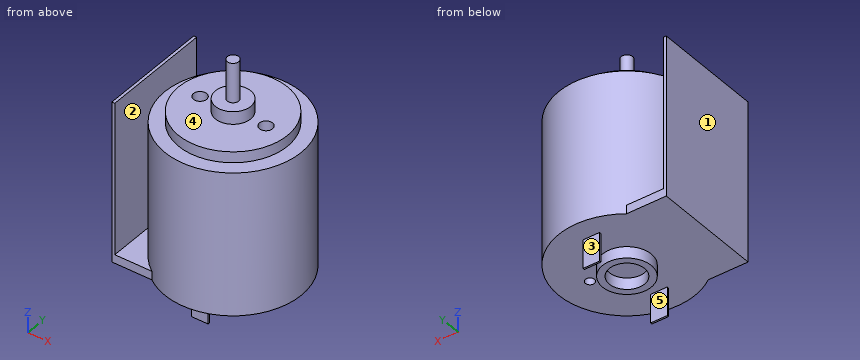
from build123d import *

# Parameters (mm, degrees)
SKETCH_2_R             = 1
EXTRUDE_1_DEPTH        = 36
SKETCH_2_4_R           = 3.075
SKETCH_2_4_R_2         = 1
EXTRUDE_2_DEPTH        = 29.1
EXTRUDE_3_DEPTH        = 26.9
EXTRUDE_3_DEPTH_BACK   = 2
SKETCH_2_5_R           = 4.25
SKETCH_2_5_R_2         = 3.075
SKETCH_2_6_R           = 9.5
SKETCH_2_6_R_2         = 4.25
EXTRUDE_4_DEPTH        = 26.9
SKETCH_2_7_R           = 11.9
SKETCH_2_7_R_2         = 9.5
EXTRUDE_5_DEPTH        = 25
SKETCH_5_W             = 2.9
SKETCH_5_H             = 0.3
EXTRUDE_6_DEPTH        = 5
HOLE_WIZARD_M2_2_D     = 1.6
HOLE_WIZARD_M2_2_DEPTH = 6
HOLE_WIZARD_M2_2_TIP   = 0.480688495
SKETCH_14_R            = 1.15
CUT_EXTRUDE_1_DEPTH    = 3
SKETCH_15_W            = 0.5
SKETCH_15_H            = 19.17801297
EXTRUDE_7_DEPTH        = 28
SKETCH_17_W            = 1.5
SKETCH_17_H            = 19.17801297
EXTRUDE_9_DEPTH        = 10


with BuildPart() as part:
    # Sketch 2 → Extrude 1 (new body)
    with BuildSketch(Plane.XY):
        Circle(SKETCH_2_R)
    extrude(amount=EXTRUDE_1_DEPTH)

    # Sketch 2_4 → Extrude 2 (add)
    with BuildSketch(Plane.XY):
        Circle(SKETCH_2_4_R)
        Circle(SKETCH_2_4_R_2, mode=Mode.SUBTRACT)
    extrude(amount=EXTRUDE_2_DEPTH)

    # Sketch 2_5 → Extrude 3 (add, two sides: drawn at the far end of the back side and taken through both)
    with BuildSketch(Plane.XY.offset(-EXTRUDE_3_DEPTH_BACK)):
        Circle(SKETCH_2_5_R)
        Circle(SKETCH_2_5_R_2, mode=Mode.SUBTRACT)
    extrude(amount=EXTRUDE_3_DEPTH + EXTRUDE_3_DEPTH_BACK)

    # Sketch 2_6 → Extrude 4 (add)
    with BuildSketch(Plane.XY):
        with Locations(Location((0, 0, 0), (0, 0, 180))):
            Circle(SKETCH_2_6_R)
        Circle(SKETCH_2_6_R_2, mode=Mode.SUBTRACT)
    extrude(amount=EXTRUDE_4_DEPTH)

    # Sketch 2_7 → Extrude 5 (add)
    with BuildSketch(Plane.XY):
        Circle(SKETCH_2_7_R)
        with Locations(Location((0, 0, 0), (0, 0, 180))):
            Circle(SKETCH_2_7_R_2, mode=Mode.SUBTRACT)
    extrude(amount=EXTRUDE_5_DEPTH)

    # Sketch 5 → Extrude 6 (add)
    with BuildSketch(Plane(origin=(0, 0, 0), x_dir=(-1, 0, 0), z_dir=(0, 0, -1))):
        with Locations((0, -7.656829655)):
            Rectangle(SKETCH_5_W, SKETCH_5_H)
        with Locations((0, 8.189714354)):
            Rectangle(SKETCH_5_W, SKETCH_5_H)
    extrude(amount=EXTRUDE_6_DEPTH)

    # Hole Wizard M2 _2
    with Locations(Plane(origin=(0, 0, 0), x_dir=(-1, 0, 0), z_dir=(0, 0, -1))):
        with Locations((-6.45, 0), (6.45, 0)):
            Hole(HOLE_WIZARD_M2_2_D / 2, depth=HOLE_WIZARD_M2_2_DEPTH)
            with Locations((0, 0, -(HOLE_WIZARD_M2_2_DEPTH + HOLE_WIZARD_M2_2_TIP / 2))):  # 118° drill point
                Cone(0, HOLE_WIZARD_M2_2_D / 2, HOLE_WIZARD_M2_2_TIP, mode=Mode.SUBTRACT)

    # Sketch 14 → Cut-Extrude 1 (cut)
    with BuildSketch(Plane.XY.offset(26.9)):
        with Locations((5.75, 0)):
            Circle(SKETCH_14_R)
        with Locations((-5.75, 0)):
            Circle(SKETCH_14_R)
    extrude(amount=-CUT_EXTRUDE_1_DEPTH, mode=Mode.SUBTRACT)



with BuildPart() as body_2:
    # Sketch 15 → Extrude 7 (new body)
    with BuildSketch(Plane(origin=(0, 0, 0), x_dir=(-1, 0, 0), z_dir=(0, 0, -1))):
        with Locations((13.75, 0)):
            Rectangle(SKETCH_15_W, SKETCH_15_H)
    extrude(amount=-EXTRUDE_7_DEPTH)


with BuildPart() as part_1:
    add(part.part)

    add(body_2.part)  # Extrude 9 merges body 2
    # Sketch 17 → Extrude 9 (add)
    with BuildSketch(Plane.ZY.offset(14)):
        with Locations((0.75, 0)):
            Rectangle(SKETCH_17_W, SKETCH_17_H)
    extrude(amount=-EXTRUDE_9_DEPTH)


solid = part_1.part
Geometry: final body of the model. Coordinates: model frame, mm. Face numbers are marked on the shaded views. A direction names the side the tool comes from. Round coordinates to 2 decimals unless told otherwise and drop trailing zeros. Loops run counter-clockwise (first coordinate to the right, second up) from the corner with the lowest first, then second, coordinate; pieces in that order, holes last.
Q1. Section C-C on x = -8.5. Return loops of the section in (y, z), plus the area to 3 significant figures.
Q2. Pin query (flat end, axial travel): P1, Ø5, axis at x = -7, z = 25, coming from the +Y side; P2, Ø1.4, axis at x = 0, z = -1.5, coming from the -Y side; P3, Ø3, axis at y = -7.5, z = 8.5, coming from the +X side. Return the tip coordinate at first contact, or that it passes through.
Q3. Section A-A on z = 19.5. Return loops of the section in (x, y), plus the area to 3 significant figures.
Q4. Material intervals for L1, parallel to X at y = 0, z = 2.75; L2, parallel to Y at x = 0, z = -1 (3 decimals); L3, parallel to Z at x = -5.5, y = -6, sorted ascending.
Q5. Access query for the marked faces 1, 2, 3, 4 and 5. Directions: +Z, -Z, +X, -X, +Y, -Y. A direction counts if a zero-diameter tool reaches every point of the face in a straight line with its end or side. Return the directions, or none.
Evaluation:
1. outline: (-9.59, 0) - (9.59, 0) - (9.59, 1.5) - (8.33, 1.5) - (8.33, 25) - (4.24, 25) - (4.24, 26.9) - (-4.24, 26.9) - (-4.24, 25) - (-8.33, 25) - (-8.33, 1.5) - (-9.59, 1.5) - close
1. area: 436 mm2
2. P1: stops at y = 11.02
2. P2: stops at y = -7.81
2. P3: stops at x = 10.28
3. outline: (-14, -9.59) - (-13.5, -9.59) - (-13.5, 9.59) - (-14, 9.59) - close; circle Ø23.8 at (0, 0)
3. area: 454 mm2
4. L1: x = -14 to -13.5, -11.9 to -7.25, -5.65 to 5.65, 7.25 to 11.9
4. L2: y = -7.807 to -7.507, -4.25 to -3.075, 3.075 to 4.25, 8.04 to 8.34
4. L3: z = 0 to 26.9
5. face 1: +Z, -Z, -X, +Y, -Y
5. face 2: +Z, +Y, -Y
5. face 3: -Z, +X, -X, +Y
5. face 4: +Z
5. face 5: -Z, +X, -X
